Drawing for the job (mm, zero at the part's lowest x, y, z). A direction names the side the tool comes from. Coordinates: 2 decimals unless noted, no trailing zeros. Order: outer loops, then holes, each group sorted by start corner. A loop starts at its lowest first (then second) coordinate and runs counter-clockwise, first axis right, second up.
1) Tool access for the marked faces 4, 5 and 6: list every direction of +Z, -Z, +X, -X, +Y, -Y with a clear straight run to the whole face (end or side of a thin tool).
2) Mould opens along Z. For the marked faces 1, 2 and 3 say: +Z half, -Z half, draft (parallel to the pull), parting line (faces both ways), or undercut.
3) Cut at C-C (z = 31). List the corners of the cut face in (x, y), and give its area (3 significant figures).
4) Cut at D-D (x = 24.5). List the corners of the cut face in (y, z), and give its area (3 significant figures).
5) Cut at B-B (y = 110). List the corners of the cut face in (x, z).
6) Wall check: L1, parallel to Z at x = 266.5, y = 12; L2, parallel to X at y = 156.5, z = 293; L3, parallel to Y at x = 22, z = 195. Give the ranges that are in metal, low to high.
7) Cut at A-A (z = 92). List the corners of the cut face in (x, y), and give its area (3 significant figures).
8) Pin check, flat tip, straight feed: pin 1 Ø7.5 at (x, z) = (313.5, 192) entering from -Y. Stop position of the tip, or through.
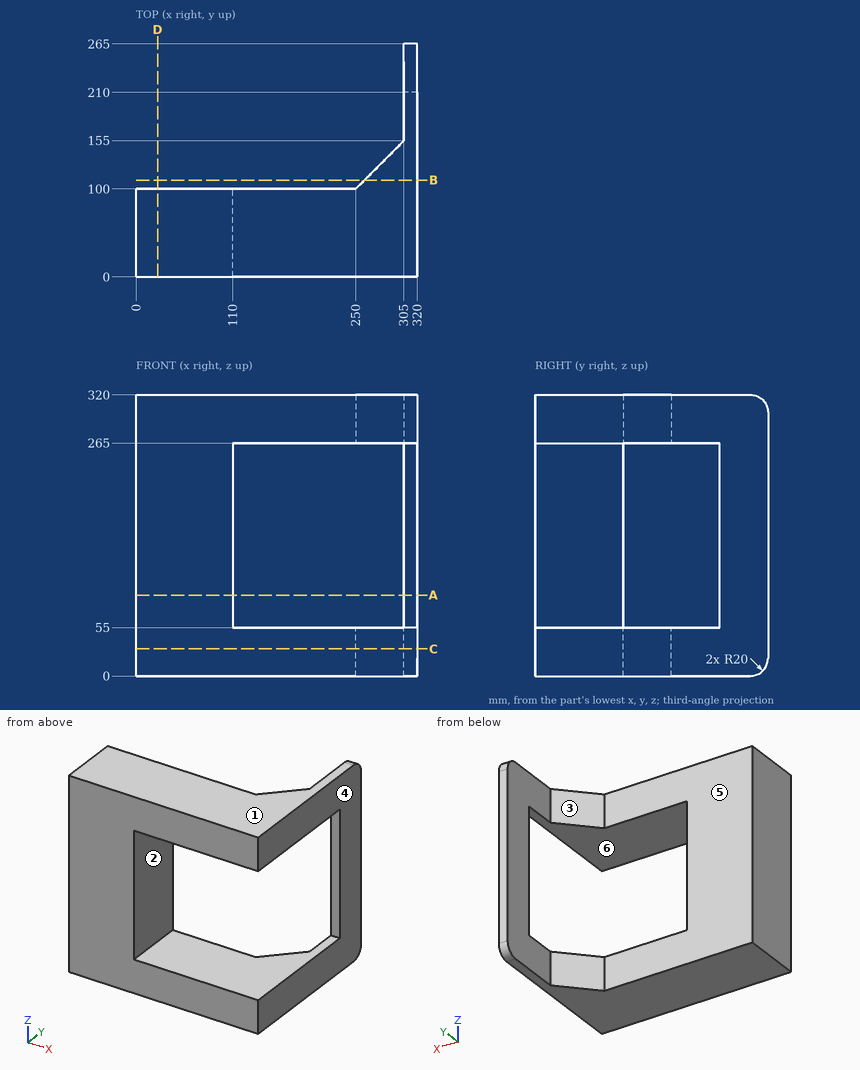
Geometry check:
1. face 4: +Z, -Z, +X, +Y, -Y
1. face 5: +Z, -Z, -X, +Y
1. face 6: +X, -Y
2. face 1: +Z half
2. face 2: undercut
2. face 3: draft
3. outline: (0, 0) - (320, 0) - (320, 265) - (305, 265) - (305, 155) - (250, 100) - (0, 100) - close
3. area: 36,000 mm2
4. outline: (0, 0) - (100, 0) - (100, 320) - (0, 320) - close
4. area: 32,000 mm2
5. outline: (260, 0) - (320, 0) - (320, 55) - (260, 55) - close; (260, 265) - (320, 265) - (320, 320) - (260, 320) - close
6. L1: z = 0 to 55, 265 to 320
6. L2: x = 305 to 320
6. L3: y = 0 to 100
7. outline: (0, 0) - (110, 0) - (110, 100) - (0, 100) - close; (305, 210) - (320, 210) - (320, 265) - (305, 265) - close
7. area: 11,800 mm2
8. pin 1: stops at y = 210
